```python
from build123d import *

# Parameters (mm, degrees)
F0_W     = 27.5
F0_H     = 55
F0_R     = 2.5
F0_H_2   = 20.950978
F1_DEPTH = 7
F2_W     = 55
F2_H     = 75.950978
F3_DEPTH = 5
F4_DEPTH = 1.5


with BuildPart() as f1:
    # F0 (on Front) → F1 (new body)
    with BuildSketch(Plane.XZ):
        with Locations((-47.613798, 47.863281)):
            Rectangle(F0_W, F0_H)
        with Locations((-56.909575, 70.300661)):
            Circle(F0_R, mode=Mode.SUBTRACT)
        Polygon((-33.863798, 20.363281), (-61.363798, 20.363281), (-61.363798, -34.636719), (48.636202, -34.636719), (48.636202, 20.363281), (21.136202, 20.363281), (21.136202, -0.587697), (-6.363798, -0.587697), (-33.863798, -0.587697), align=None)
        with Locations((-56.909575, -29.699339)):
            Circle(F0_R, mode=Mode.SUBTRACT)
        with Locations((43.090425, -29.699339)):
            Circle(F0_R, mode=Mode.SUBTRACT)
        with Locations((34.886202, 47.863281)):
            Rectangle(F0_W, F0_H)
        with Locations((43.090425, 70.300661)):
            Circle(F0_R, mode=Mode.SUBTRACT)
        Polygon((-6.363798, 75.363281), (-33.863798, 75.363281), (-33.863798, 20.363281), (-6.363798, 20.363281), (-6.363798, 32.674998), (-10.402054, 34.54878), (-10.841582, 39.465519), (-6.803326, 42.30453), (-6.363798, 42.100586), align=None)
        Polygon((21.136202, 75.363281), (-6.363798, 75.363281), (-6.363798, 42.100586), (-2.325542, 40.226804), (-1.886014, 35.310065), (-5.92427, 32.471054), (-6.363798, 32.674998), (-6.363798, 20.363281), (21.136202, 20.363281), align=None)
        with Locations((-20.113798, 9.887792)):
            Rectangle(F0_W, F0_H_2)
        with Locations((7.386202, 9.887792)):
            Rectangle(F0_W, F0_H_2)
        with BuildLine():
            Line((-2.325542, 40.226804), (-6.363798, 42.100586))
            Line((-6.363798, 42.100586), (-6.363798, 39.387792))
            ThreePointArc((-6.363798, 39.387792), (-4.949584, 38.802006), (-4.363798, 37.387792))
            ThreePointArc((-4.363798, 37.387792), (-4.949584, 35.973578), (-6.363798, 35.387792))
            Line((-6.363798, 35.387792), (-6.363798, 32.674998))
            Line((-6.363798, 32.674998), (-5.92427, 32.471054))
            Line((-5.92427, 32.471054), (-1.886014, 35.310065))
            Line((-1.886014, 35.310065), (-2.325542, 40.226804))
        make_face()
        with BuildLine():
            Line((-6.363798, 39.387792), (-6.363798, 42.100586))
            Line((-6.363798, 42.100586), (-6.803326, 42.30453))
            Line((-6.803326, 42.30453), (-10.841582, 39.465519))
            Line((-10.841582, 39.465519), (-10.402054, 34.54878))
            Line((-10.402054, 34.54878), (-6.363798, 32.674998))
            Line((-6.363798, 32.674998), (-6.363798, 35.387792))
            ThreePointArc((-6.363798, 35.387792), (-8.363798, 37.387792), (-6.363798, 39.387792))
        make_face()
    extrude(amount=F1_DEPTH)

    # F2 (on face) → F3 (cut)
    with BuildSketch(Plane.XZ.offset(7)):
        with Locations((-6.363798, 37.387792)):
            Rectangle(F2_W, F2_H)
    extrude(amount=-F3_DEPTH, mode=Mode.SUBTRACT)

    # F0 (on Front) → F4 (cut)
    with BuildSketch(Plane.XZ):
        with BuildLine():
            Line((-2.325542, 40.226804), (-6.363798, 42.100586))
            Line((-6.363798, 42.100586), (-6.363798, 39.387792))
            ThreePointArc((-6.363798, 39.387792), (-4.949584, 38.802006), (-4.363798, 37.387792))
            ThreePointArc((-4.363798, 37.387792), (-4.949584, 35.973578), (-6.363798, 35.387792))
            Line((-6.363798, 35.387792), (-6.363798, 32.674998))
            Line((-6.363798, 32.674998), (-5.92427, 32.471054))
            Line((-5.92427, 32.471054), (-1.886014, 35.310065))
            Line((-1.886014, 35.310065), (-2.325542, 40.226804))
        make_face()
        with BuildLine():
            Line((-6.363798, 39.387792), (-6.363798, 42.100586))
            Line((-6.363798, 42.100586), (-6.803326, 42.30453))
            Line((-6.803326, 42.30453), (-10.841582, 39.465519))
            Line((-10.841582, 39.465519), (-10.402054, 34.54878))
            Line((-10.402054, 34.54878), (-6.363798, 32.674998))
            Line((-6.363798, 32.674998), (-6.363798, 35.387792))
            ThreePointArc((-6.363798, 35.387792), (-8.363798, 37.387792), (-6.363798, 39.387792))
        make_face()
    extrude(amount=F4_DEPTH, mode=Mode.SUBTRACT)


solid = f1.part
```
Geometry check sheet. Reference: the model listing, model coordinates, mm. A direction names the side the tool comes from. Give positions to 0.01 mm unless a question says otherwise; leave off trailing zeros. Write each loop counter-clockwise with the first axis right and the second up, starting at its lowest first coordinate (ties: lowest second). Pieces come first, ordered by that corner, then holes. Notation, with made-up numbers: (49, -21) - (73, -21) arc R32 cw to (73, 7) - close; hole circle Ø4 at (-11.75, 83.5). An arc over 180 degrees is marked (long way). Use a Markdown table: item, result.
Q1. Section check C-C, the plane x = -30. Enter the section's corners in (y, z), then the cut area to 3 significant figures.
Computed:
| item | result |
|---|---|
| outline | (-7, -34.64) - (0, -34.64) - (0, 75.36) - (-2, 75.36) - (-2, -0.59) - (-7, -0.59) - close |
| area | 390 mm² |
Q2. Thickness scan on L1, parallel to X at y = -3, z = 39.5; L2, parallel to Z at x = -8.5, y = -4; L3, parallel to Y at x = -27.5, z = 32. Record the ranges inside material, lowest first. Write a range as [from, to].
Computed:
| item | result |
|---|---|
| L1 | x = [-61.36, -33.86], [21.14, 48.64] |
| L2 | z = [-34.64, -0.59] |
| L3 | y = [-2, 0] |
Q3. Go/stop test with flat-tipped pins: P1, Ø2, axis at x = 17.5, z = 20.5, coming from the -Y side; P2, Ø2.5, axis at x = 6.5, y = -5, coming from the +Z side. Record where each tip stops, or that it passes through.
Computed:
| item | result |
|---|---|
| P1 | stops at y = -2 |
| P2 | stops at z = -0.59 |
Q4. Section check B-B, the plane y = -5. Enter the section's corners in (x, z), then the cut area to 3 significant figures.
Computed:
| item | result |
|---|---|
| outline | (-61.36, -34.64) - (48.64, -34.64) - (48.64, 75.36) - (21.14, 75.36) - (21.14, -0.59) - (-33.86, -0.59) - (-33.86, 75.36) - (-61.36, 75.36) - close; hole circle Ø5 at (-56.91, -29.7); hole circle Ø5 at (-56.91, 70.3); hole circle Ø5 at (43.09, -29.7); hole circle Ø5 at (43.09, 70.3) |
| area | 7,840 mm² |
Q5. Draft check along X on faces 1 (the face through (-7, -7, -3)), 2 (the face through (48.636, -3, 20)), 3 (the face through (42.76, -3.45, 72.78)). Enter one of: pulls with the +X half, pulls with the -X half, needs draft (parallel to the pull), parting line crosses it, or undercut.
Computed:
| item | result |
|---|---|
| face 1 | needs draft |
| face 2 | pulls with the +X half |
| face 3 | undercut |
Q6. Section check A-A, the plane z = 66. Enter the section's corners in (x, y).
Computed:
| item | result |
|---|---|
| outline | (-61.36, -7) - (-33.86, -7) - (-33.86, -2) - (21.14, -2) - (21.14, -7) - (48.64, -7) - (48.64, 0) - (-61.36, 0) - close |
Q7. Set-up check for faces 4 (the face through (-33.864, -5, 37)), 5 (the face through (-59.407, -3.451, -29.589)), 6 (the face through (-3.933, -0.74, 33.871)): record each of +Z, -Z, +X, -X, +Y, -Y from which the full face is reachable in a straight line by a thin tool's end or side.
Computed:
| item | result |
|---|---|
| face 4 | +Z, -Y |
| face 5 | +Y, -Y |
| face 6 | +Y |
